CAD build for the part. Positions are in the model's coordinates, mm. Face numbers are marked on the shaded views. Give positions to 0.01 mm unless a question says otherwise; leave off trailing zeros. Order: outer loops, then holes, each group sorted by start corner. A loop starts at its lowest first (then second) coordinate and runs counter-clockwise, first axis right, second up. Notation, with made-up numbers: M 26,41 L 37,41 A24 cw 37,67 Z; hole C -13.5,23.25 d1. An arc over 180 degrees is marked long. Put each result on its own line as item: value. Start each with the question number.
1) Drill centre lines: line 1 (X direction, y = 7.25, z = 23); line 2 (X direction, y = 7.5, z = 21); line 3 (Z direction, x = 7.5, y = 1.5). Where is each one in solid material? Low to high. Write a range as [from, to].
2) Two-plate mould, pull along Z, no slides. Class the marked faces 1, 2 and 3: released by +Z, released by -Z, zero draft, split by the parting line, or undercut.
3) Cut at A-A (y = 19). Write the cut outline in (x, z).
4) Cut at C-C (x = -14). Write the cut outline in (y, z), and give its area (3 significant figures).
5) Cut at B-B (z = 32). Write the cut outline in (x, y), and give its area (3 significant figures).
6) Pin check, flat tip, straight feed: pin 1 (1.5 mm diameter, centred on x = 15, y = 5.5, fed in from +Z). Stop position of the tip, or through.
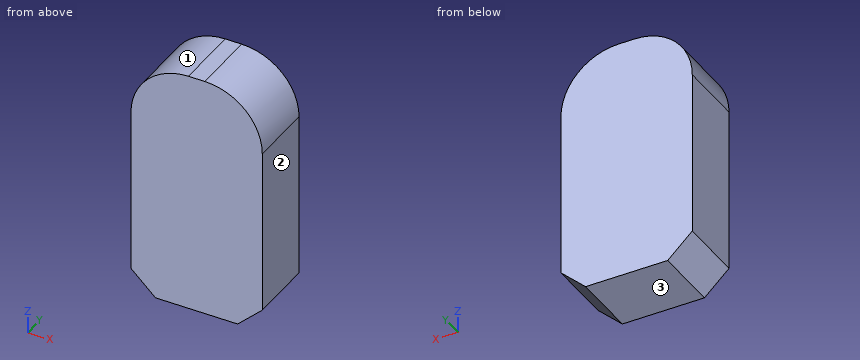
```python
from build123d import *

# Parameters (mm, degrees)
BOSS_EXTRUDE2_DEPTH = 20


with BuildPart() as part:
    # Sketch1 → Boss-Extrude2 (new body)
    with BuildSketch(Plane(origin=(0, 0, 0), x_dir=(1, 0, 0), z_dir=(0, 1, 0))):
        with BuildLine():
            Line((-12.5, 37.5), (12.5, 37.5))
            Line((12.5, 37.5), (20, 30.5))
            Line((20, 30.5), (20, -20))
            ThreePointArc((20, -20), (14.874368671, -32.374368671), (2.5, -37.5))
            Line((2.5, -37.5), (-2.5, -37.5))
            ThreePointArc((-2.5, -37.5), (-14.874368671, -32.374368671), (-20, -20))
            Line((-20, -20), (-20, 30.5))
            Line((-20, 30.5), (-12.5, 37.5))
        make_face()
    extrude(amount=BOSS_EXTRUDE2_DEPTH)


solid = part.part
```
Solution:
1. line 1: [-19.74, 19.74]
1. line 2: [-19.97, 19.97]
1. line 3: [-37.5, 36.77]
2. face 1: released by +Z
2. face 2: zero draft
2. face 3: released by -Z
3. outline: M -20,-30.5 L -12.5,-37.5 L 12.5,-37.5 L 20,-30.5 L 20,20 A17.5 ccw 2.5,37.5 L -2.5,37.5 A17.5 ccw -20,20 Z
4. outline: M 0,-36.1 L 20,-36.1 L 20,33.19 L 0,33.19 Z
4. area: 1,390 mm²
5. outline: M -15.24,0 L 15.24,0 L 15.24,20 L -15.24,20 Z
5. area: 610 mm²
6. pin 1: z = 32.97
